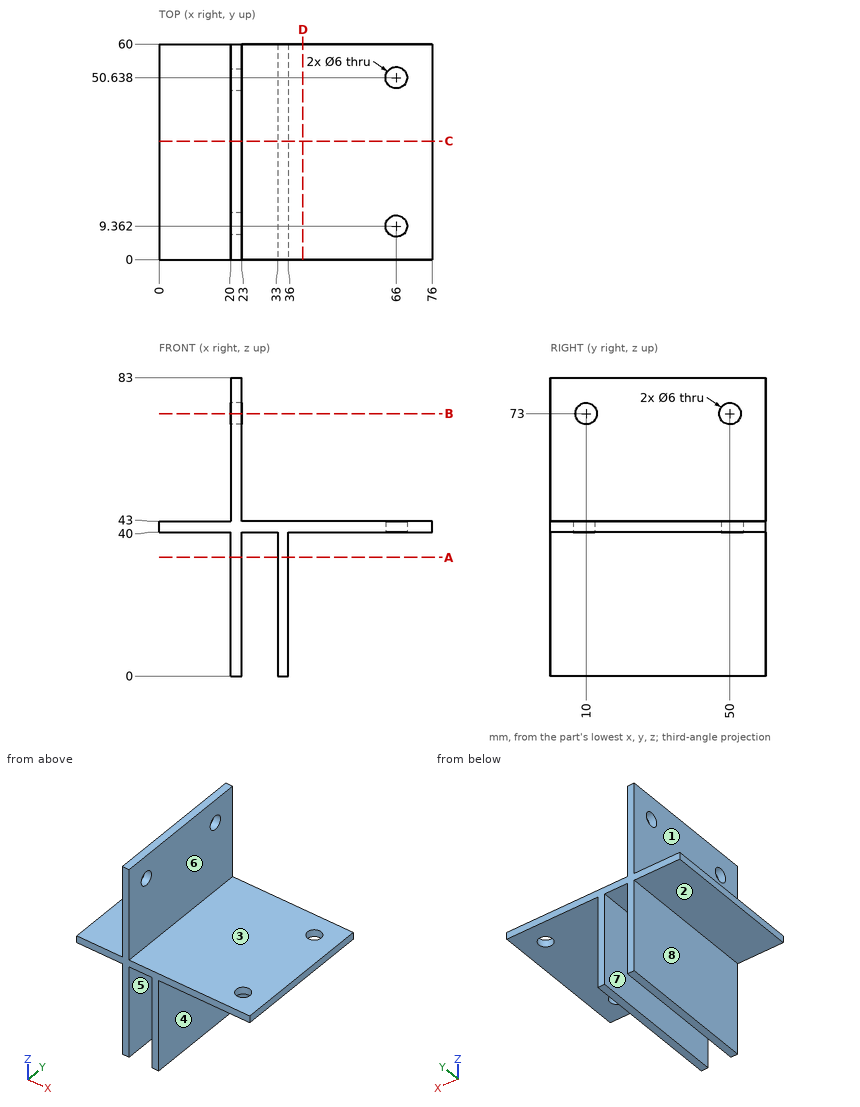
For this review, use the dimensioned drawing (mm, ordinates from the lowest corner) and the shaded views. A direction names the side the tool comes from. Round coordinates to 2 decimals unless told otherwise and drop trailing zeros. Write each loop counter-clockwise with the first axis right and the second up, starting at its lowest first coordinate (ties: lowest second). Pieces come first, ordered by that corner, then holes. Notation, with made-up numbers: M -11.5,12 L 9.5,12 A30 cw 9.5,46 Z; hole C 15.5,58.25 d5. An arc over 180 degrees is marked long. Use CSV: the item, a comma, the result in double quotes. Start each with the question number.
(1) We need section C-C, the plane y = 33. State the section outline as (x, z) points.
(2) Tool access review of the marked faces 1, 2, 3, 4 and 5: name each direction out of +Z, -Z, +X, -X, +Y, -Y from which nothing blocks a thin tool from reaching the whole face with its end or side.
(3) Clearance check with flat-ended pins moving along their axes: P1, Ø6, axis at x = 10.5, y = 41, coming from the -Z side; P2, Ø5, axis at x = 66, y = 9.36, coming from the +Z side; P3, Ø12, axis at y = 20.5, z = 64.5, coming from the +X side; P4, Ø1, axis at y = 12.5, z = 67.5, coming from the -X side. State where each tip first meets the part, or that it passes through.
(4) The part is to be moulded in two halves that separate along X. For the marked faces 6, 7 and 8, say which applies: +X half, -X half, draft (parallel to the pull), parting line (faces both ways), or undercut.
(5) We need section D-D, the plane x = 40. State the section outline as (y, z) points.
(6) We need section B-B, the plane z = 73. State the section outline as (x, y) points.
(7) For line 1 along Y through (x, z) = (66, 41.95); line 2 along X through (y, z) = (20, 8.5); line 3 along X through (y, z) = (6, 53.5), list the stretches that pass through material, from the lowest coordinate up.
(8) We need section A-A, the plane z = 33. State the section outline as (x, y) points.
Findings:
1,outline,"M 0,40 L 20,40 L 20,0 L 23,0 L 23,40 L 33,40 L 33,0 L 36,0 L 36,40 L 76,40 L 76,43 L 23,43 L 23,83 L 20,83 L 20,43 L 0,43 Z"
2,face 1,"+Z, -X, +Y, -Y"
2,face 2,"-Z, -X, +Y, -Y"
2,face 3,"+Z, +X, +Y, -Y"
2,face 4,"-Z, +X, +Y, -Y"
2,face 5,"-Z, +Y, -Y"
3,P1,"z = 40"
3,P2,"through"
3,P3,"x = 23"
3,P4,"x = 20"
4,face 6,"+X half"
4,face 7,"undercut"
4,face 8,"-X half"
5,outline,"M 0,40 L 60,40 L 60,43 L 0,43 Z"
6,outline,"M 20,0 L 23,0 L 23,7 L 20,7 Z; M 20,13 L 23,13 L 23,47 L 20,47 Z; M 20,53 L 23,53 L 23,60 L 20,60 Z"
7,line 1,"0 to 6.36, 12.36 to 47.64, 53.64 to 60"
7,line 2,"20 to 23, 33 to 36"
7,line 3,"20 to 23"
8,outline,"M 20,0 L 23,0 L 23,60 L 20,60 Z; M 33,0 L 36,0 L 36,60 L 33,60 Z"
